Here's how the part is built. I have some questions about the finished solid (model axes, mm). A direction names the side the tool comes from. Round coordinates to 2 decimals unless told otherwise and drop trailing zeros. Write each loop counter-clockwise with the first axis right and the second up, starting at its lowest first coordinate (ties: lowest second). Pieces come first, ordered by that corner, then holes. Notation, with made-up numbers: (-32.75, 43) - (13.25, 43) arc R18 cw to (13.25, 54) - close; hole circle Ø2 at (-6, -4.75). An arc over 180 degrees is marked (long way). Write item = value, one per line. Start each with the question number.
Item 1: If we section it at B-B (y = -4.5): Please give me the cut outline in (x, z), and give its area (3 significant figures).
Item 2: If I drill on line 1 along Z through (x, y) = (6, -11); line 2 along Y through (x, z) = (8, -12.5); line 3 along Y through (x, z) = (3.25, -2.5), over which ranges is the centre line in solid material (lowest first)? Write a range as [from, to].
Item 3: For P1, Ø8, axis at x = 9, z = -9.5, coming from the -Y side; P2, Ø1, axis at x = 11.5, z = -17.5, coming from the -Y side; P3, Ø1, axis at x = 7, z = -14, coming from the +Y side, each with a flat end and sliding along its axis, tell me the tip position at first contact or that it passes through.
Item 4: If we section it at A-A (z = -11.25): Please give me the cut outline in (x, y), and give its area (3 significant figures).
Item 5: Thinking about a two-plate mould opening in Z: for faces 1 (the face through (5, -6, -4)), 2 (the face through (7, 5, -3.048)), 3 (the face through (0, 1, -10)), which applies, pulls with the +Z half, pulls with the -Z half, needs draft (parallel to the pull), parting line crosses it, or undercut?
Item 6: If we section it at D-D (x = 11): Please give me the cut outline in (y, z), and give its area (3 significant figures).
Item 7: Which directions (+Z, -Z, +X, -X, +Y, -Y) give clear straight access to the entire face, cutting with the end or side of a thin tool? Please do faces 4 (the face through (7, 8, -13)), 5 (the face through (7, 3, -12)), 6 (the face through (9, 0, -10)).
Item 8: If we section it at C-C (x = 9.5): Please give me the cut outline in (y, z), and give its area (3 significant figures).
```python
from build123d import *

# Parameters (mm, degrees)
SKETCH1_W               = 20
SKETCH1_H               = 9.5
BOSS_EXTRUDE1_DEPTH     = 15
CUT_EXTRUDE1_DEPTH      = 27.744158241
CUT_EXTRUDE1_DEPTH_BACK = 27.744158241
SKETCH4_R               = 1.25
BOSS_EXTRUDE3_DEPTH     = 4


with BuildPart() as part:
    # Sketch1 → Boss-Extrude1 (new body)
    with BuildSketch(Plane(origin=(0, 0, 0), x_dir=(0, 0, -1), z_dir=(1, 0, 0))):
        with Locations((10, 4.75)):
            Rectangle(SKETCH1_W, SKETCH1_H)
    extrude(amount=BOSS_EXTRUDE1_DEPTH)

    # Sketch2 → Cut-Extrude1 (cut, two sides: drawn at the far end of the back side and taken through both)
    with BuildSketch(Plane(origin=(15, 0, 0), x_dir=(0, 0, -1), z_dir=(1, 0, 0)).offset(-CUT_EXTRUDE1_DEPTH_BACK)):
        Polygon((20, 3), (3.047520991, 3), (3.047520991, 6.5), (13, 6.5), (13, 9.5), (20, 9.5), (20, 6.3375), align=None)
    extrude(amount=CUT_EXTRUDE1_DEPTH + CUT_EXTRUDE1_DEPTH_BACK, mode=Mode.SUBTRACT)

    # Sketch4 → Boss-Extrude3 (add)
    with BuildSketch(Plane.XY):
        with BuildLine():
            Line((0, 0), (0, -12))
            ThreePointArc((0, -12), (3.202154051, -15.202154051), (6.404308102, -12))
            Line((6.404308102, -12), (12, 0))
            Line((12, 0), (0, 0))
        make_face()
        with Locations((3.202154051, -12)):
            Circle(SKETCH4_R, mode=Mode.SUBTRACT)
    boss_extrude3 = extrude(amount=-BOSS_EXTRUDE3_DEPTH)

    # Mirror1: Boss-Extrude3 across plane
    add(boss_extrude3.mirror(Plane.XY.offset(-10)))


solid = part.part
```
Reply:
q1.outline = (0, -20) - (9.9, -20) - (9.9, -16) - (0, -16) - close; (0, -4) - (9.9, -4) - (9.9, 0) - (0, 0) - close
q1.area = 79.2 mm2
q2.line_1 = [-20, -16], [-4, 0]
q2.line_2 = [0, 3], [6.5, 9.5]
q2.line_3 = [-15.2, -13.25], [-10.75, 9.5]
q3.P1 = 0
q3.P2 = -2.14
q3.P3 = 3
q4.outline = (0, 0) - (15, 0) - (15, 3) - (0, 3) - close; (0, 6.5) - (15, 6.5) - (15, 9.5) - (0, 9.5) - close
q4.area = 90.0 mm2
q5.face_1 = undercut
q5.face_2 = pulls with the -Z half
q5.face_3 = needs draft
q6.outline = (-2.14, -20) - (3, -20) - (3, -3.05) - (6.5, -3.05) - (6.5, -13) - (9.5, -13) - (9.5, 0) - (-2.14, 0) - (-2.14, -4) - (0, -4) - (0, -16) - (-2.14, -16) - close
q6.area = 127 mm2
q7.face_4 = -Z, +X, -X, +Y
q7.face_5 = -Z, +X, -X
q7.face_6 = +X, -Y
q8.outline = (-5.36, -20) - (3, -20) - (3, -3.05) - (6.5, -3.05) - (6.5, -13) - (9.5, -13) - (9.5, 0) - (-5.36, 0) - (-5.36, -4) - (0, -4) - (0, -16) - (-5.36, -16) - close
q8.area = 153 mm2
